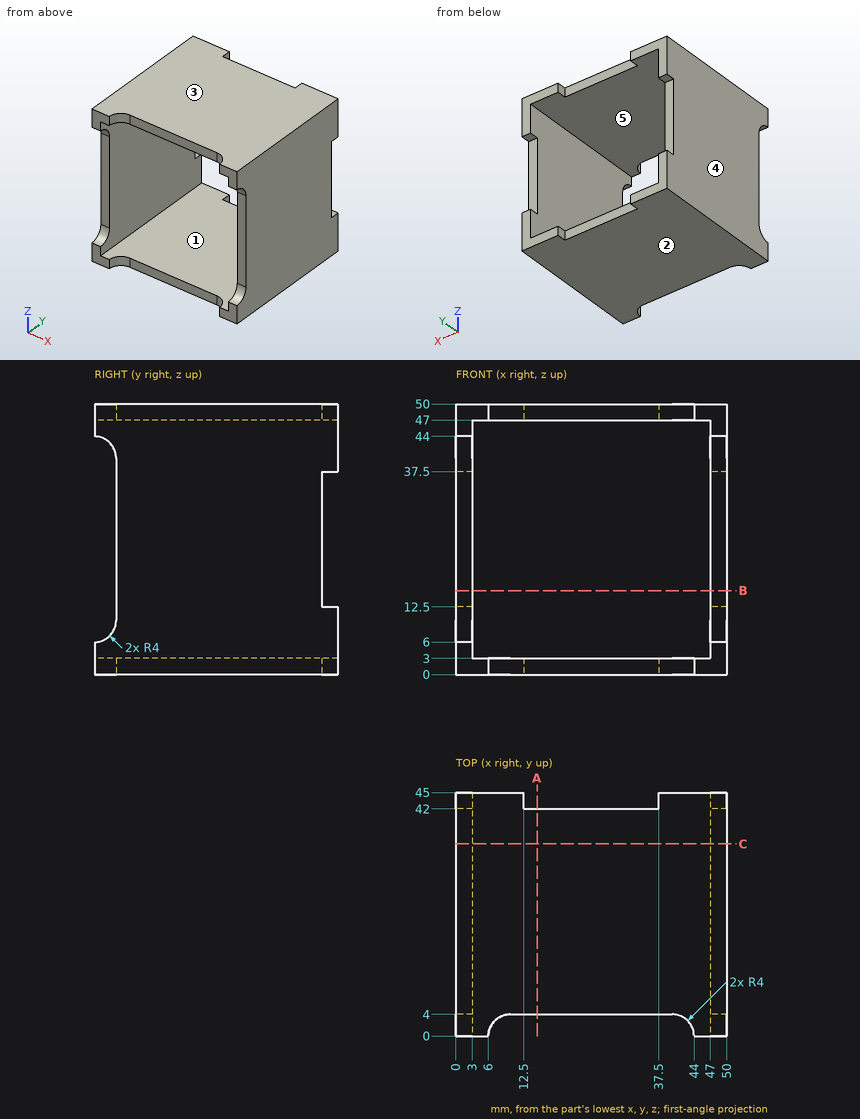
Verification items for this drawing (mm, ordinates from the low corner). A direction names the side the tool comes from. Coordinates: 2 decimals unless noted, no trailing zeros. Loops run counter-clockwise (first coordinate to the right, second up) from the corner with the lowest first, then second, coordinate; pieces in that order, holes last. Notation, with made-up numbers: (-38.75, -9.75) - (-20.75, -9.75) arc R30 ccw to (-20.75, 19.25) - close; hole circle Ø4 at (53, 6.5). An arc over 180 degrees is marked (long way). One line per item, written item: value. Start each with the question number.
(1) Cross-section at B-B on z = 15.5. Enter the section's corners in (x, y).
(2) Mould release check, pull along X, two halves, no side actions. Record for the marked faces 3, 4 and 5: released by +X, released by -X, zero draft, split by the parting line, or undercut.
(3) Depth check by flat-ended pin: P1, Ø1.5, axis at x = 48.5, z = 30, coming from the +Y side; P2, Ø10, axis at x = 38.5, z = 14, coming from the +Y side; P3, Ø1.5, axis at x = 22.5, z = 1, coming from the -Y side. Enter the tip coordinate at first touch or a pass-through.
(4) Material ranges on line 1 (X direction, y = 20.5, z = 9); line 2 (Y direction, x = 2, z = 13), recorded low to high. Write a range as [from, to].
(5) Cross-section at C-C on y = 35.5. Enter the section's corners in (x, z).
(6) Tool access check on the marked faces 1 and 2. Record the directions out of +Z, -Z, +X, -X, +Y, -Y that give a thin tool (end or side, any length) a straight path to the whole face; none if there is none.
(7) Cross-section at A-A on x = 15. Enter the section's corners in (y, z), plus the area to 3 significant figures.
Results below:
1. outline: (0, 4) - (3, 4) - (3, 42) - (0, 42) - close; (47, 4) - (50, 4) - (50, 42) - (47, 42) - close
2. face 3: zero draft
2. face 4: released by -X
2. face 5: undercut
3. P1: stops at y = 42
3. P2: passes through
3. P3: stops at y = 4
4. line 1: x = [0, 3], [47, 50]
4. line 2: y = [4, 42]
5. outline: (0, 0) - (50, 0) - (50, 50) - (0, 50) - close; hole (3, 3) - (47, 3) - (47, 47) - (3, 47) - close
6. face 1: +Y, -Y
6. face 2: -Z, +X, -X, +Y, -Y
7. outline: (4, 0) - (42, 0) - (42, 3) - (4, 3) - close; (4, 47) - (42, 47) - (42, 50) - (4, 50) - close
7. area: 228 mm2
